The figure shows three views and two pictorial views of one solid part (mm, origin at its lowest corner). Answer the questions. A direction names the side the tool comes from. Round coordinates to 2 decimals unless told otherwise and drop trailing zeros. Loops run counter-clockwise (first coordinate to the right, second up) from the corner with the lowest first, then second, coordinate; pieces in that order, holes last. Notation, with made-up numbers: (20, 19) -> (48, 19) arc R19 ccw to (48, 30) -> close; hole circle Ø8 at (67, 42.5). An arc over 180 degrees is marked (long way). Use a Markdown table: item, result. Add a question column.
Q1. Which of the six approach directions +Z, -Z, +X, -X, +Y, -Y give full straight-line access (tool end or side, diameter ignored) to the marked faces 1, 2 and 3?
Q2. Section C-C on z = 16.5 is taken. Give the vertices of the cut face in (x, y), then the cut area to 3 significant figures.
Q3. Section A-A on x = 11.5 is taken. Give the vertices of the cut face in (y, z).
Q4. Given pin 1 Ø7.5 at (x, z) = (8, 23.5) entering from -Y; pin 2 Ø7.5 at (x, z) = (6, 18.5) entering from +Y, each flat-ended and moving along its own axis, determine where each tip first touches the part or whether it passes through.
Q5. Section D-D on z = 40 is taken. Give the vertices of the cut face in (x, y), then the cut area to 3 significant figures.
Q6. Section B-B on y = 65 is taken. Give the vertices of the cut face in (x, z).
Q7. For a pull along Z with two mould halves and no side action, classify the marked faces 4, 5, 6 and 7 as released by +Z, released by -Z, zero draft, split by the parting line, or undercut.
Q8. Consider line 1 (Z direction, x = 8.75, y = 10); line 2 (Y direction, x = 14, z = 14.5); line 3 (Z direction, x = 12.75, y = 65.5). Determine where each line is inside the solid, lowest interval first.
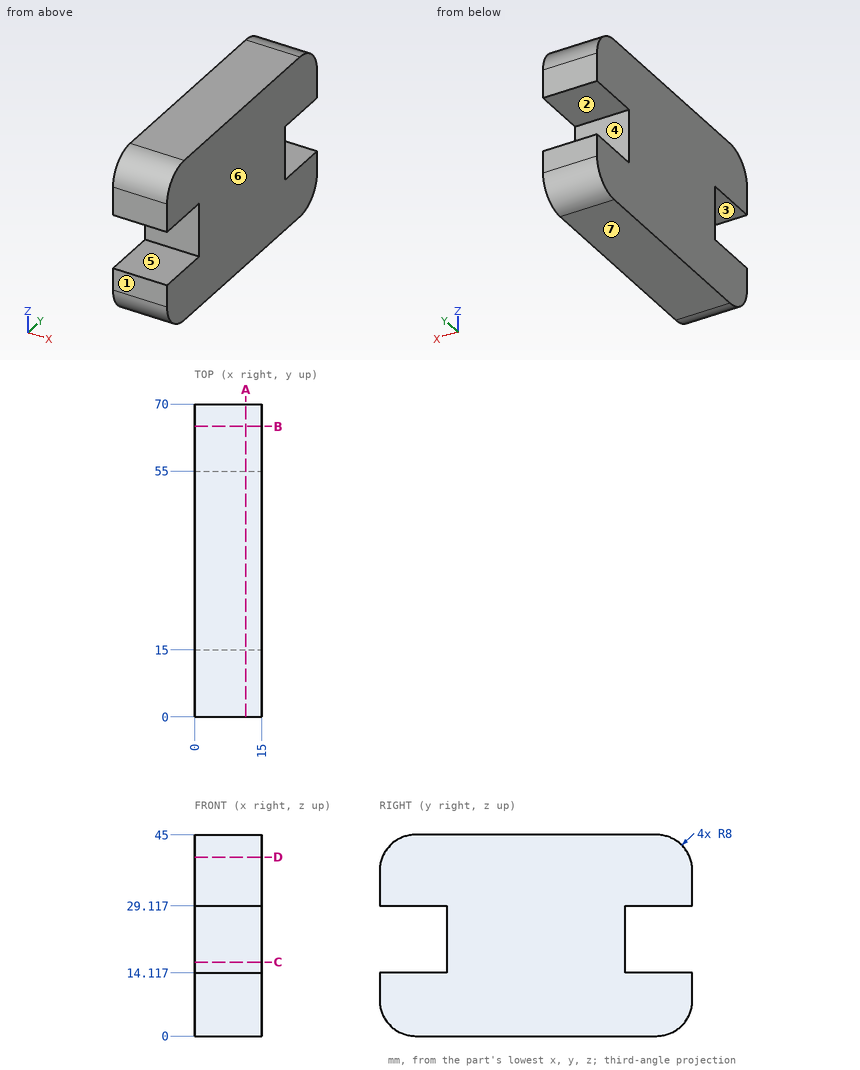
Checked values:
| question | item | result |
|---|---|---|
| 1 | face 1 | +Z, -Z, +X, -X, -Y |
| 1 | face 2 | +X, -X, +Y |
| 1 | face 3 | +X, -X, -Y |
| 2 | outline | (0, 15) -> (15, 15) -> (15, 55) -> (0, 55) -> close |
| 2 | area | 600 mm2 |
| 3 | outline | (0, 8) arc R8 ccw to (8, 0) -> (62, 0) arc R8 ccw to (70, 8) -> (70, 14.12) -> (55, 14.12) -> (55, 29.12) -> (70, 29.12) -> (70, 37) arc R8 ccw to (62, 45) -> (8, 45) arc R8 ccw to (0, 37) -> (0, 29.12) -> (15, 29.12) -> (15, 14.12) -> (0, 14.12) -> close |
| 4 | pin 1 | stops at y = 15 |
| 4 | pin 2 | stops at y = 55 |
| 5 | outline | (0, 0.58) -> (15, 0.58) -> (15, 69.42) -> (0, 69.42) -> close |
| 5 | area | 1,030 mm2 |
| 6 | outline | (0, 0.58) -> (15, 0.58) -> (15, 14.12) -> (0, 14.12) -> close; (0, 29.12) -> (15, 29.12) -> (15, 44.42) -> (0, 44.42) -> close |
| 7 | face 4 | undercut |
| 7 | face 5 | undercut |
| 7 | face 6 | zero draft |
| 7 | face 7 | released by -Z |
| 8 | line 1 | z = 0 to 14.12, 29.12 to 45 |
| 8 | line 2 | y = 15 to 55 |
| 8 | line 3 | z = 0.81 to 14.12, 29.12 to 44.19 |
